```python
from build123d import *

# Parameters (mm, degrees)
SKETCH_1_R          = 3
EXTRUDE_1_DEPTH     = 10
CUT_EXTRUDE_1_DEPTH = 10
CUT_EXTRUDE_2_DEPTH = 10


with BuildPart() as part:
    # 草图1 → 凸台-拉伸1 (new body)
    with BuildSketch(Plane.XY):
        Circle(SKETCH_1_R)
    extrude(amount=EXTRUDE_1_DEPTH)

    # 草图2 → 切除-拉伸1 (cut)
    with BuildSketch(Plane.XY.offset(10)):
        with BuildLine():
            Line((1.120267825, 1.005), (-1.120267825, 1.005))
            ThreePointArc((-1.120267825, 1.005), (0, -1.505), (1.120267825, 1.005))
        make_face()
    extrude(amount=-CUT_EXTRUDE_1_DEPTH, mode=Mode.SUBTRACT)

    # 草图3 → 切除-拉伸2 (cut)
    with BuildSketch(Plane(origin=(0, 0, 0), x_dir=(-1, 0, 0), z_dir=(0, 0, -1))):
        with BuildLine():
            Line((-1.65074983, 2.505), (1.65074983, 2.505))
            ThreePointArc((1.65074983, 2.505), (0, 3), (-1.65074983, 2.505))
        make_face()
    extrude(amount=-CUT_EXTRUDE_2_DEPTH, mode=Mode.SUBTRACT)


solid = part.part
```
Geometry: final body of the model. Coordinates: model frame, mm. Round coordinates to 2 decimals unless told otherwise and drop trailing zeros. Loops run counter-clockwise (first coordinate to the right, second up) from the corner with the lowest first, then second, coordinate; pieces in that order, holes last. Notation, with made-up numbers: (42.25, -0.5) -> (47.25, -0.5) arc R8 ccw to (47.25, 13.5) -> close; hole circle Ø4 at (7.5, 21). An arc over 180 degrees is marked (long way). Use one line per item in the form item = value.
Item 1: Draft query along X for faces 1 (the flat face through (0, 2.505, 5)), 2 (the cylindrical face through (0, -3, 5)), 3 (the cylindrical face through (-0.048, -1.504, 5.07)). Return one class per face: released by +X, released by -X, zero draft, split by the parting line, or undercut.
Evaluation:
face_1 = zero draft
face_2 = split by the parting line
face_3 = undercut
Item 2: Cut plane A-A on y = 0. Output: boundary loops of the cut face in (x, z) (3 decimals).
Evaluation:
outline = (-3, 0) -> (-1.505, 0) -> (-1.505, 10) -> (-3, 10) -> close; (1.505, 0) -> (3, 0) -> (3, 10) -> (1.505, 10) -> close
Item 3: Cut plane B-B on x = 0. Output: boundary loops of the cut face in (y, z) (3 decimals).
Evaluation:
outline = (-3, 0) -> (-1.505, 0) -> (-1.505, 10) -> (-3, 10) -> close; (1.005, 0) -> (2.505, 0) -> (2.505, 10) -> (1.005, 10) -> close
Item 4: Cut plane D-D on y = 1.15. Output: boundary loops of the cut face in (x, z), then the cut area to 3 significant figures.
Evaluation:
outline = (-2.77, 0) -> (2.77, 0) -> (2.77, 10) -> (-2.77, 10) -> close
area = 55.4 mm2
Item 5: Cut plane C-C on z = 6. Output: boundary loops of the cut face in (x, y) (3 decimals).
Evaluation:
outline = (-1.651, 2.505) arc R3 ccw (long way) to (1.651, 2.505) -> close; hole (-1.12, 1.005) arc R1.505 ccw (long way) to (1.12, 1.005) -> close
Item 6: Material intervals for probe 1 along X at (y, z) = (0, 6.5) (3 decimals); probe 2 along Y at (x, z) = (0, 4.5) (3 decimals); probe 3 along Y at (x, z) = (1, 3) (3 decimals), sorted ascending.
Evaluation:
probe_1 = -3 to -1.505, 1.505 to 3
probe_2 = -3 to -1.505, 1.005 to 2.505
probe_3 = -2.828 to -1.125, 1.005 to 2.505
